Can you work these out from the drawing? Everything is in mm from the part's minimum corner. Coordinates: 2 decimals unless noted, no trailing zeros. Order: outer loops, then holes, each group sorted by start corner. A loop starts at its lowest first (then second) coordinate and runs counter-clockwise, first axis right, second up. Notation, with made-up numbers: (-33, -16.75) -> (-22, -16.75) arc R19 ccw to (-22, 18.25) -> close; hole circle Ø9 at (-5, 67.5). An arc over 180 degrees is marked (long way). Use a Markdown table: item, result. Add a question column.
1) If we section it at A-A (x = 128): Write out the boundary of the cut face in (y, z), plus the area to 3 significant figures.
2) If I drill on L1, parallel to Z at x = 267, y = 0.85; L2, parallel to X at y = 0.85, z = 8; L3, parallel to Z at x = 92, y = 1.4, over which ranges is the centre line in solid material (lowest first)? Write a range as [from, to].
3) If we section it at C-C (x = 52): Write out the boundary of the cut face in (y, z).
4) If we section it at B-B (z = 72.5): Write out the boundary of the cut face in (x, y) (3 decimals).
5) If we section it at D-D (z = 96.5): Write out the boundary of the cut face in (x, y) (3 decimals), plus the area to 3 significant figures.
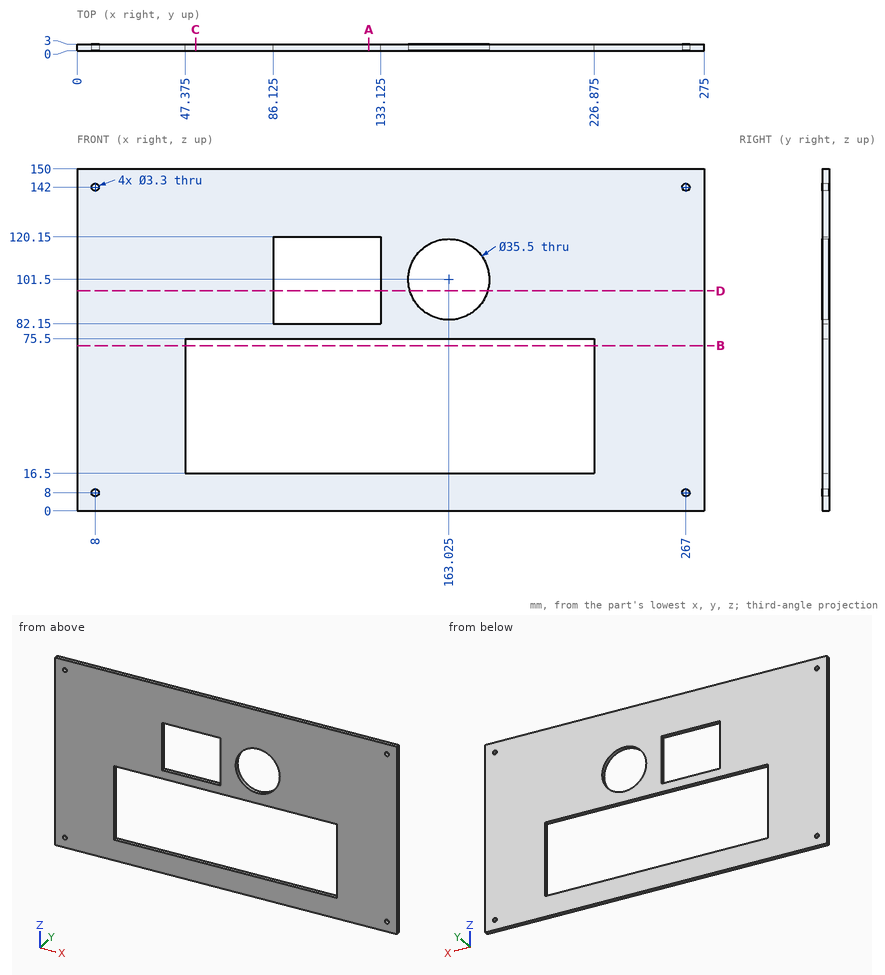
Answer sheet:
| question | item | result |
|---|---|---|
| 1 | outline | (0, 0) -> (3, 0) -> (3, 16.5) -> (0, 16.5) -> close; (0, 75.5) -> (3, 75.5) -> (3, 82.15) -> (0, 82.15) -> close; (0, 120.15) -> (3, 120.15) -> (3, 150) -> (0, 150) -> close |
| 1 | area | 159 mm2 |
| 2 | L1 | [0, 6.35], [9.65, 140.35], [143.65, 150] |
| 2 | L2 | [0, 6.35], [9.65, 265.35], [268.65, 275] |
| 2 | L3 | [0, 16.5], [75.5, 82.15], [120.15, 150] |
| 3 | outline | (0, 0) -> (3, 0) -> (3, 16.5) -> (0, 16.5) -> close; (0, 75.5) -> (3, 75.5) -> (3, 150) -> (0, 150) -> close |
| 4 | outline | (0, 0) -> (47.375, 0) -> (47.375, 3) -> (0, 3) -> close; (226.875, 0) -> (275, 0) -> (275, 3) -> (226.875, 3) -> close |
| 5 | outline | (0, 0) -> (86.125, 0) -> (86.125, 3) -> (0, 3) -> close; (133.125, 0) -> (145.994, 0) -> (145.994, 3) -> (133.125, 3) -> close; (180.056, 0) -> (275, 0) -> (275, 3) -> (180.056, 3) -> close |
| 5 | area | 582 mm2 |
